from build123d import *

# Parameters (mm, degrees)
SKETCH_1_W          = 10
SKETCH_1_H          = 10
EXTRUDE_1_DEPTH     = 38
CUT_EXTRUDE_1_DEPTH = 22
SKETCH_4_R          = 2.1
CUT_EXTRUDE_2_DEPTH = 22


with BuildPart() as part:
    # 草图1 → 凸台-拉伸1 (new body)
    with BuildSketch(Plane.XY):
        with Locations((5, 5)):
            Rectangle(SKETCH_1_W, SKETCH_1_H)
    extrude(amount=EXTRUDE_1_DEPTH)

    # 草图3 → 切除-拉伸1 (cut)
    with BuildSketch(Plane(origin=(0, 10, 0), x_dir=(1, 0, 0), z_dir=(0, 1, 0))):
        with BuildLine():
            ThreePointArc((7.1, -8), (6.48492424, -6.51507576), (5, -5.9))
            Line((5, -5.9), (5, -10.1))
            ThreePointArc((5, -10.1), (6.48492424, -9.48492424), (7.1, -8))
        make_face()
        with BuildLine():
            Line((5, -10.1), (5, -5.9))
            ThreePointArc((5, -5.9), (2.9, -8), (5, -10.1))
        make_face()
        with BuildLine():
            ThreePointArc((7.1, -30), (6.48492424, -28.51507576), (5, -27.9))
            Line((5, -27.9), (5, -32.1))
            ThreePointArc((5, -32.1), (6.48492424, -31.48492424), (7.1, -30))
        make_face()
        with BuildLine():
            Line((5, -32.1), (5, -27.9))
            ThreePointArc((5, -27.9), (2.9, -30), (5, -32.1))
        make_face()
    extrude(amount=-CUT_EXTRUDE_1_DEPTH, mode=Mode.SUBTRACT)

    # 草图4 → 切除-拉伸2 (cut)
    with BuildSketch(Plane(origin=(10, 0, 0), x_dir=(0, 0, -1), z_dir=(1, 0, 0))):
        with Locations(Location((-25, 5, 0), (0, 0, 90))):
            Circle(SKETCH_4_R)
        with Locations(Location((-13, 5, 0), (0, 0, 90))):
            Circle(SKETCH_4_R)
    extrude(amount=-CUT_EXTRUDE_2_DEPTH, mode=Mode.SUBTRACT)


solid = part.part
Geometry: final body of the model. Coordinates: model frame, mm. Give positions to 0.01 mm unless a question says otherwise; leave off trailing zeros. Write each loop counter-clockwise with the first axis right and the second up, starting at its lowest first coordinate (ties: lowest second). Pieces come first, ordered by that corner, then holes. Notation, with made-up numbers: M 81,73 L 140,73 A33 ccw 140,111 Z; hole C 72,12.25 d2. An arc over 180 degrees is marked long. Answer in a Markdown table with one row per item. Add a question column.
(1) Section D-D on y = 1. Return loops of the section in (x, z).
(2) Section A-A on y = 5. Return loops of the section in (x, z), and give its area (3 significant figures).
(3) Ray query, line 1 (Z direction, x = 7.25, y = 3.75); line 2 (Z direction, x = 4.75, y = 5); line 3 (Z direction, x = 5.75, y = 3.5). Return the intervals inside material, ascending.
(4) Section B-B on x = 3.25. Return loops of the section in (y, z).
(5) First-contact query: pin 1 (2.5 mm diameter, centred on y = 5, z = 25, fed in from -X). Flat tip, straight axial feed; report the tip coordinate or a pass-through.
(6) Section C-C on z = 25. Return loops of the section in (x, y), and give its area (3 significant figures).
(7) Mould query, pull axis Z, two halves, no side actions, for faces 1 (the flat face through (5, 5, 38)), 2 (the cylindrical face through (5.07, 2.9, 13.09)), 3 (the cylindrical face through (5.07, 6.13, 26.77)), 4 (the flat face through (10, 5, 19)). Classes: +Z half, -Z half, draft (parallel to the pull), parting line (faces both ways), or undercut.
Result set:
| question | item | result |
|---|---|---|
| 1 | outline | M 0,0 L 10,0 L 10,38 L 0,38 Z; hole C 5,8 d4.2; hole C 5,30 d4.2 |
| 2 | outline | M 0,0 L 10,0 L 10,10.9 L 0,10.9 Z; M 0,15.1 L 10,15.1 L 10,22.9 L 0,22.9 Z; M 0,27.1 L 10,27.1 L 10,38 L 0,38 Z; hole C 5,8 d4.2; hole C 5,30 d4.2 |
| 2 | area | 268 mm^2 |
| 3 | line 1 | z = 0 to 11.31, 14.69 to 23.31, 26.69 to 38 |
| 3 | line 2 | z = 0 to 5.91, 10.09 to 10.9, 15.1 to 22.9, 27.1 to 27.91, 32.09 to 38 |
| 3 | line 3 | z = 0 to 6.04, 9.96 to 11.53, 14.47 to 23.53, 26.47 to 28.04, 31.96 to 38 |
| 4 | outline | M 0,0 L 10,0 L 10,6.84 L 0,6.84 Z; M 0,9.16 L 10,9.16 L 10,28.84 L 0,28.84 Z; M 0,31.16 L 10,31.16 L 10,38 L 0,38 Z; hole C 5,13 d4.2; hole C 5,25 d4.2 |
| 5 | pin 1 | passes through |
| 6 | outline | M 0,0 L 10,0 L 10,2.9 L 0,2.9 Z; M 0,7.1 L 10,7.1 L 10,10 L 0,10 Z |
| 6 | area | 58.0 mm^2 |
| 7 | face 1 | +Z half |
| 7 | face 2 | undercut |
| 7 | face 3 | undercut |
| 7 | face 4 | draft |
